For this review, use the dimensioned drawing (mm, ordinates from the lowest corner) and the shaded views. A direction names the side the tool comes from. Give positions to 0.01 mm unless a question says otherwise; leave off trailing zeros. Loops run counter-clockwise (first coordinate to the right, second up) from the corner with the lowest first, then second, coordinate; pieces in that order, holes last. Notation, with made-up numbers: (80, 71.25) - (95, 71.25) arc R31 cw to (95, 110.25) - close; hole circle Ø7 at (69.5, 48). An arc over 180 degrees is marked (long way). Write each question's results on one line, items separated by ' | '.
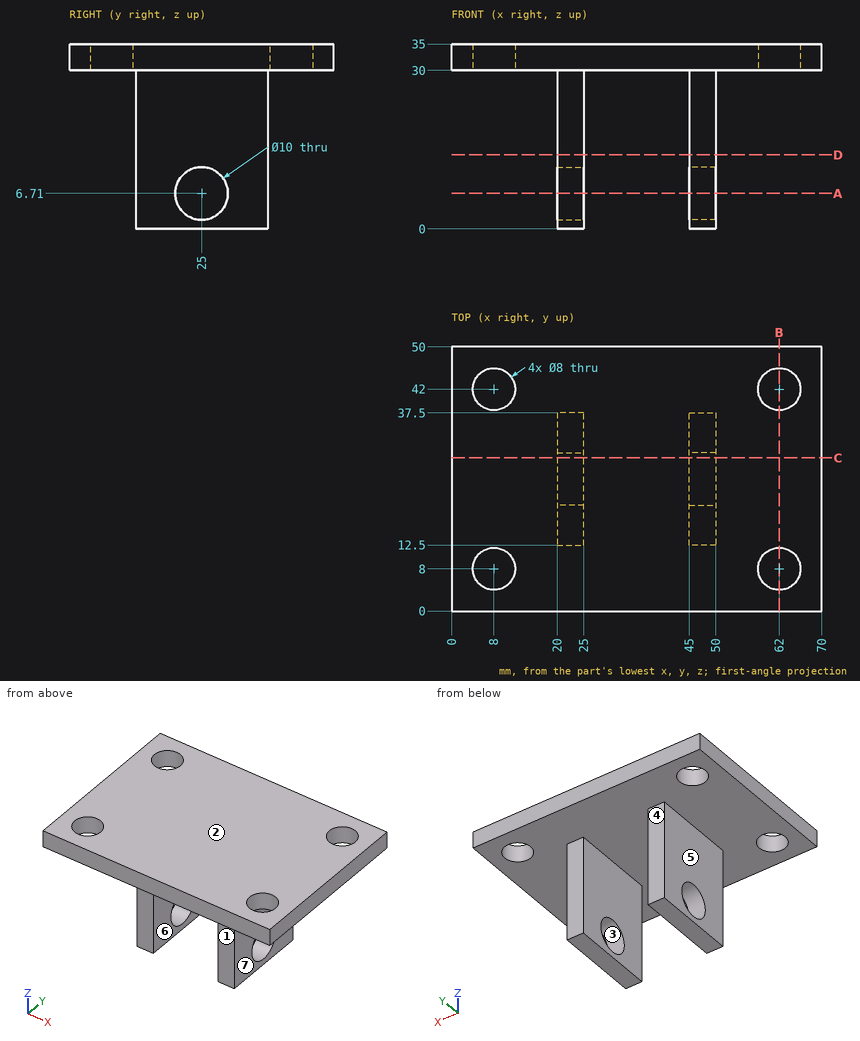
Item 1: Wall thickness on probe 1 along X at (y, z) = (8, 32.1); probe 2 along Y at (x, z) = (8, 32.4); probe 3 along X at (y, z) = (24, 25): over which ranges is each line inside the solid? List them lowest first.
Output values:
probe 1: x = 0 to 4, 12 to 58, 66 to 70 | probe 2: y = 0 to 4, 12 to 38, 46 to 50 | probe 3: x = 20 to 25, 45 to 50
Item 2: We need section D-D on z = 14. Give the boundary of the cut face in (x, y).
Output values:
outline: (20, 12.5) - (25, 12.5) - (25, 37.5) - (20, 37.5) - close; (45, 12.5) - (50, 12.5) - (50, 37.5) - (45, 37.5) - close
Item 3: Tool access review of the marked faces 4, 5, 6 and 7: name each direction out of +Z, -Z, +X, -X, +Y, -Y from which nothing blocks a thin tool from reaching the whole face with its end or side.
Output values:
face 4: -Z, +X, -X, +Y | face 5: -Z, -X, +Y, -Y | face 6: -Z, +Y, -Y | face 7: -Z, +X, +Y, -Y
Item 4: We need section B-B on x = 62. Give the boundary of the cut face in (y, z).
Output values:
outline: (0, 30) - (4, 30) - (4, 35) - (0, 35) - close; (12, 30) - (38, 30) - (38, 35) - (12, 35) - close; (46, 30) - (50, 30) - (50, 35) - (46, 35) - close
Item 5: Draft analysis for pull direction Z (two halves, no side actions). For the marked faces 1, 2 and 3, state which applies: +Z half, -Z half, draft (parallel to the pull), parting line (faces both ways), or undercut.
Output values:
face 1: draft | face 2: +Z half | face 3: undercut
Item 6: We need section A-A on z = 6.71. Give the boundary of the cut face in (x, y), then the cut area to 3 significant figures.
Output values:
outline: (20, 12.5) - (25, 12.5) - (25, 20) - (20, 20) - close; (20, 30) - (25, 30) - (25, 37.5) - (20, 37.5) - close; (45, 12.5) - (50, 12.5) - (50, 20) - (45, 20) - close; (45, 30) - (50, 30) - (50, 37.5) - (45, 37.5) - close | area: 150 mm²
Item 7: Clearance check with flat-ended pins moving along their axes: P1, Ø1.5, axis at x = 23, z = 19.5, coming from the -Y side; P2, Ø5.5, axis at x = 48, z = 21.5, coming from the +Y side; P3, Ø1.5, axis at x = 52.5, z = 10, coming from the +Y side; P4, Ø20, axis at y = 24, z = 9, coming from the -X side. State where each tip first meets the part, or that it passes through.
Output values:
P1: stops at y = 12.5 | P2: stops at y = 37.5 | P3: passes through | P4: stops at x = 20
Item 8: We need section C-C on y = 29. Give the boundary of the cut face in (x, z), then the cut area to 3 significant figures.
Output values:
outline: (0, 30) - (20, 30) - (20, 9.71) - (25, 9.71) - (25, 30) - (45, 30) - (45, 9.71) - (50, 9.71) - (50, 30) - (70, 30) - (70, 35) - (0, 35) - close; (20, 0) - (25, 0) - (25, 3.71) - (20, 3.71) - close; (45, 0) - (50, 0) - (50, 3.71) - (45, 3.71) - close | area: 590 mm²
